```python
from build123d import *

# Parameters (mm, degrees)
F0_W     = 58
F0_H     = 38
F1_DEPTH = 3
F0_W_2   = 60
F0_H_2   = 40
F2_DEPTH = 10
F3_R     = 1.5


with BuildPart() as f1:
    # F0 (on Top) → F1 (new body)
    with BuildSketch(Plane.XY):
        Rectangle(F0_W, F0_H)
    extrude(amount=F1_DEPTH)

    # F0 (on Top) → F2 (join)
    with BuildSketch(Plane.XY):
        Rectangle(F0_W_2, F0_H_2)
        Rectangle(F0_W, F0_H, mode=Mode.SUBTRACT)
    extrude(amount=F2_DEPTH)

    # F3
    f3_edges = [f1.edges().sort_by_distance(p)[0] for p in [
        (-30, -20, 5),
        (30, -20, 5),
        (30, 20, 5),
        (-30, 20, 5),
    ]]
    fillet(f3_edges, radius=F3_R)


solid = f1.part
```
Here's how the part is built. I have some questions about the finished solid (model axes, mm). A direction names the side the tool comes from. Give positions to 0.01 mm unless a question says otherwise; leave off trailing zeros. Order: outer loops, then holes, each group sorted by start corner. A loop starts at its lowest first (then second) coordinate and runs counter-clockwise, first axis right, second up. Notation, with made-up numbers: (-12, 31.5) - (7, 31.5) arc R10 cw to (7, 36.5) - close; hole circle Ø10 at (50, 12.5). An arc over 180 degrees is marked (long way). Answer as a JSON object with one key per item and string values. Group by question number.
Item 1: For P1, Ø11.5, axis at x = 14, y = -8, coming from the +Z side, with a flat end and sliding along its axis, tell me the tip position at first contact or that it passes through.
Item 2: If we mould it in two halves opening along X, with no side actions, what happens to faces 1 (the flat face through (0, 0, 0)), 2 (the flat face through (-29, 0, 6)), 3 (the cylindrical face through (-29.57, 19.55, 5.07)), 4 (the flat face through (0, -19, 6))? For each: pulls with the +X half, pulls with the -X half, needs draft (parallel to the pull), parting line crosses it, or undercut.
Item 3: Please list where these lines run through material, in increasing order: probe 1 along X at (y, z) = (-10, 7.75); probe 2 along Y at (x, z) = (14.5, 4); probe 3 along Z at (x, y) = (9, 9.5).
Item 4: Which directions (+Z, -Z, +X, -X, +Y, -Y) give clear straight access to the entire face, cutting with the end or side of a thin tool? Please do faces 5 (the flat face through (30, 0, 5)), 6 (the flat face through (0, 0, 3)).
Item 5: If we section it at A-A on z = 4.25: Please give me the cut outline in (x, y).
Item 6: If we section it at C-C on x = -16: Please give me the cut outline in (y, z).
Item 7: If we section it at B-B on y = 5: Please give me the cut outline in (x, z), and give its area (3 significant figures).
Result set:
{
 "1": {"P1": "z = 3"},
 "2": {"face 1": "needs draft", "face 2": "undercut", "face 3": "pulls with the -X half", "face 4": "undercut"},
 "3": {"probe 1": "-30 to -29, 29 to 30", "probe 2": "-20 to -19, 19 to 20", "probe 3": "0 to 3"},
 "4": {"face 5": "+Z, -Z, +X, +Y, -Y", "face 6": "+Z"},
 "5": {"outline": "(-30, -18.5) arc R1.5 ccw to (-28.5, -20) - (28.5, -20) arc R1.5 ccw to (30, -18.5) - (30, 18.5) arc R1.5 ccw to (28.5, 20) - (-28.5, 20) arc R1.5 ccw to (-30, 18.5) - close; hole (-29, -19) - (29, -19) - (29, 19) - (-29, 19) - close"},
 "6": {"outline": "(-20, 0) - (20, 0) - (20, 10) - (19, 10) - (19, 3) - (-19, 3) - (-19, 10) - (-20, 10) - close"},
 "7": {"outline": "(-30, 0) - (30, 0) - (30, 10) - (29, 10) - (29, 3) - (-29, 3) - (-29, 10) - (-30, 10) - close", "area": "194 mm²"}
}
